Geometry check sheet. Reference: the model listing, model coordinates, mm. Face numbers are marked on the shaded views. A direction names the side the tool comes from. Coordinates: 2 decimals unless noted, no trailing zeros. Loops run counter-clockwise (first coordinate to the right, second up) from the corner with the lowest first, then second, coordinate; pieces in that order, holes last. Notation, with made-up numbers: (74, 71.25) - (123, 71.25) arc R18 ccw to (123, 88.25) - close; hole circle Ø9 at (75.5, 44). An arc over 180 degrees is marked (long way). One line per item, written item: value.
from build123d import *

# Parameters (mm, degrees)
SKETCH1_R             = 5
BOSS_EXTRUDE1_DEPTH   = 1
BOSS_EXTRUDE1_2_DEPTH = 1
BOSS_EXTRUDE2_DEPTH   = 3
F_4_CLEARANCE_HOLE1_D = 3.2639
CUT_EXTRUDE1_DEPTH    = 1


with BuildPart() as part:
    # Sketch1 → Boss-Extrude1 (new body)
    with BuildSketch(Plane(origin=(0, 0, 0), x_dir=(1, 0, 0), z_dir=(0, 1, 0))):
        with Locations(Location((-15, 0, 0), (0, 0, 270))):
            Circle(SKETCH1_R)
    extrude(amount=BOSS_EXTRUDE1_DEPTH)



with BuildPart() as body_2:
    # Sketch1 → Boss-Extrude1 2 (new body)
    with BuildSketch(Plane(origin=(0, 0, 0), x_dir=(1, 0, 0), z_dir=(0, 1, 0))):
        with Locations(Location((15, 0, 0), (0, 0, 270))):
            Circle(SKETCH1_R)
    extrude(amount=BOSS_EXTRUDE1_2_DEPTH)


with BuildPart() as part_1:
    add(part.part)

    add(body_2.part)  # Boss-Extrude2 merges body 2
    # Sketch2 → Boss-Extrude2 (add)
    with BuildSketch(Plane(origin=(0, 1, 0), x_dir=(1, 0, 0), z_dir=(0, 1, 0))):
        with BuildLine():
            Line((-15, -5), (15, -5))
            ThreePointArc((15, -5), (20, 0), (15, 5))
            Line((15, 5), (-15, 5))
            ThreePointArc((-15, 5), (-20, 0), (-15, -5))
        make_face()
    extrude(amount=BOSS_EXTRUDE2_DEPTH)

    # #4 Clearance Hole1 (through all)
    with Locations(Plane(origin=(0, 4, 0), x_dir=(1, 0, 0), z_dir=(0, 1, 0))):
        with Locations((-15, 0), (15, 0)):
            Hole(F_4_CLEARANCE_HOLE1_D / 2)

    # Sketch5 → Cut-Extrude1 (cut)
    with BuildSketch(Plane.XZ):
        with BuildLine():
            Line((12.5, 3), (12.5, 6))
            Line((12.5, 6), (9.5, 6))
            ThreePointArc((9.5, 6), (7.378679656, 5.121320344), (6.5, 3))
            Line((6.5, 3), (6.5, 0))
            Line((6.5, 0), (9.5, 0))
            ThreePointArc((9.5, 0), (11.621320344, 0.878679656), (12.5, 3))
        make_face()
        with BuildLine():
            Line((-12.5, 3), (-12.5, 6))
            Line((-12.5, 6), (-9.5, 6))
            ThreePointArc((-9.5, 6), (-7.378679656, 5.121320344), (-6.5, 3))
            Line((-6.5, 3), (-6.5, 0))
            Line((-6.5, 0), (-9.5, 0))
            ThreePointArc((-9.5, 0), (-11.621320344, 0.878679656), (-12.5, 3))
        make_face()
    extrude(amount=-CUT_EXTRUDE1_DEPTH, mode=Mode.SUBTRACT)


solid = part_1.part
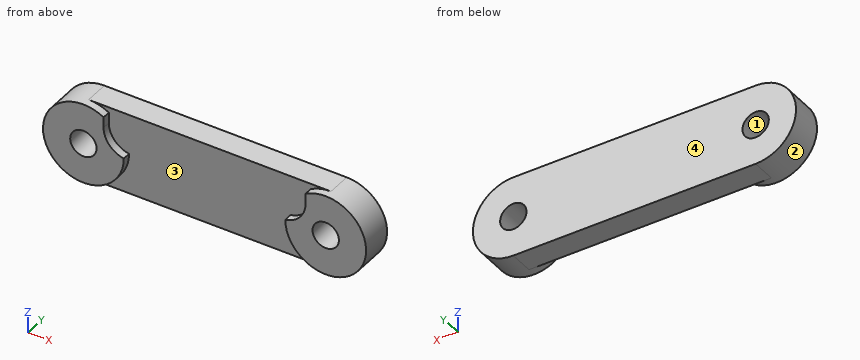
(1) Cross-section at A-A on y = 3.5. Record the cut outline in (x, z), and give its area (3 significant figures).
Reply:
outline: (-15, -5) - (15, -5) arc R5 ccw to (15, 5) - (-15, 5) arc R5 ccw to start; hole circle Ø3.26 at (-15, 0); hole circle Ø3.26 at (15, 0)
area: 362 mm2
(2) Go/stop test with flat-tipped pins: pin 1 Ø2 at (x, z) = (15, 0) entering from +Y (1 decimal); pin 2 Ø0.8 at (y, z) = (0.5, 3.5) entering from -X; pin 3 Ø3 at (x, z) = (-6.5, 0.5) entering from -Y. Record where each tip stops, or that it passes through.
Reply:
pin 1: through
pin 2: x = -18.92
pin 3: y = 1
(3) Release check for a two-part mould opening along X. For the marked faces 3 and 4 record: pulls with the +X half, pulls with the -X half, needs draft (parallel to the pull), parting line crosses it, or undercut.
Reply:
face 3: undercut
face 4: needs draft
(4) Cross-section at B-B on z = 2. Record the cut outline in (x, y), and give its area (3 significant figures).
Reply:
outline: (-19.58, 0) - (-12.33, 0) - (-12.33, 1) - (12.33, 1) - (12.33, 0) - (19.58, 0) - (19.58, 4) - (-19.58, 4) - close
area: 132 mm2
(5) Cross-section at D-D on z = -4.5. Record the cut outline in (x, y), and give its area (3 significant figures).
Reply:
outline: (-17.18, 0) - (-12.82, 0) - (-12.82, 1) - (12.82, 1) - (12.82, 0) - (17.18, 0) - (17.18, 4) - (-17.18, 4) - close
area: 112 mm2
(6) Cross-section at C-C on x = 2. Record the cut outline in (y, z), and give its area (3 significant figures).
Reply:
outline: (1, -5) - (4, -5) - (4, 5) - (1, 5) - close
area: 30.0 mm2
(7) Material ranges on probe 1 along Z at (x, y) = (15, 1.6); probe 2 along Y at (x, z) = (-1.5, -4.25); probe 3 along X at (y, z) = (1.5, -0.5), recorded low to high. Write a range as from..to.
Reply:
probe 1: -5..-1.63, 1.63..5
probe 2: 1..4
probe 3: -19.97..-16.55, -13.45..13.45, 16.55..19.97
(8) Access from +Z, -Z, +X, -X, +Y, -Y to the whole of each face (thin tool, end or side, straight path). Record for the marked faces 1 and 2.
Reply:
face 1: +Y, -Y
face 2: -Y
